```python
from build123d import *

# Parameters (mm, degrees)
SKETCH1_W           = 9.2
SKETCH1_H           = 12
BOSS_EXTRUDE1_DEPTH = 5
SKETCH3_R           = 2
BOSS_EXTRUDE2_DEPTH = 0.5
SKETCH4_R           = 1.5
BOSS_EXTRUDE3_DEPTH = 9.5
CUT_EXTRUDE1_DEPTH  = 9.5
BOSS_EXTRUDE4_DEPTH = 15.5
SKETCH8_W           = 1.5
SKETCH8_H           = 2
CUT_EXTRUDE2_DEPTH  = 1.5
SKETCH9_W           = 0.4
SKETCH9_H           = 1.196619736
BOSS_EXTRUDE5_DEPTH = 1.7
SKETCH10_R          = 2.5
BOSS_EXTRUDE6_DEPTH = 1.5
SKETCH11_R          = 1.675952799
CUT_EXTRUDE3_DEPTH  = 0.5


with BuildPart() as part:
    # Sketch1 → Boss-Extrude1 (new body, symmetric)
    with BuildSketch(Plane(origin=(0, 0, 0), x_dir=(1, 0, 0), z_dir=(0, 1, 0))):
        Rectangle(SKETCH1_W, SKETCH1_H)
    extrude(amount=BOSS_EXTRUDE1_DEPTH, both=True)

    # Sketch3 → Boss-Extrude2 (add)
    with BuildSketch(Plane(origin=(4.6, 0, 0), x_dir=(0, 0, -1), z_dir=(1, 0, 0))):
        Circle(SKETCH3_R)
    extrude(amount=BOSS_EXTRUDE2_DEPTH)

    # Sketch4 → Boss-Extrude3 (add)
    with BuildSketch(Plane(origin=(5.1, 0, 0), x_dir=(0, 0, -1), z_dir=(1, 0, 0))):
        Circle(SKETCH4_R)
    extrude(amount=BOSS_EXTRUDE3_DEPTH)

    # Sketch5 → Cut-Extrude1 (cut)
    with BuildSketch(Plane(origin=(14.6, 0, 0), x_dir=(0, 0, -1), z_dir=(1, 0, 0))):
        with BuildLine():
            Line((-1.118033989, 1), (1.118033989, 1))
            ThreePointArc((1.118033989, 1), (0, 1.5), (-1.118033989, 1))
        make_face()
    extrude(amount=-CUT_EXTRUDE1_DEPTH, mode=Mode.SUBTRACT)

    # Sketch7 → Boss-Extrude4 (add)
    with BuildSketch(Plane.ZY.offset(4.6)):
        with BuildLine():
            Line((-2, -5), (2, -5))
            ThreePointArc((2, -5), (4.828427125, -3.828427125), (6, -1))
            Line((6, -1), (6, 1))
            ThreePointArc((6, 1), (4.828427125, 3.828427125), (2, 5))
            Line((2, 5), (-2, 5))
            ThreePointArc((-2, 5), (-4.828427125, 3.828427125), (-6, 1))
            Line((-6, 1), (-6, -1))
            ThreePointArc((-6, -1), (-4.828427125, -3.828427125), (-2, -5))
        make_face()
    extrude(amount=BOSS_EXTRUDE4_DEPTH)

    # Sketch8 → Cut-Extrude2 (cut)
    with BuildSketch(Plane.ZY.offset(20.1)):
        with Locations((-5.25, 0)):
            Rectangle(SKETCH8_W, SKETCH8_H)
        with Locations((5.25, 0)):
            Rectangle(SKETCH8_W, SKETCH8_H)
    extrude(amount=-CUT_EXTRUDE2_DEPTH, mode=Mode.SUBTRACT)

    # Sketch9 → Boss-Extrude5 (add)
    with BuildSketch(Plane.ZY.offset(20.1)):
        with Locations((-3.5, 0)):
            Rectangle(SKETCH9_W, SKETCH9_H)
        with Locations((3.5, 0)):
            Rectangle(SKETCH9_W, SKETCH9_H)
    extrude(amount=BOSS_EXTRUDE5_DEPTH)

    # Sketch10 → Boss-Extrude6 (add)
    with BuildSketch(Plane.ZY.offset(20.1)):
        Circle(SKETCH10_R)
    extrude(amount=BOSS_EXTRUDE6_DEPTH)

    # Sketch11 → Cut-Extrude3 (cut)
    with BuildSketch(Plane.ZY.offset(21.6)):
        Circle(SKETCH11_R)
    extrude(amount=-CUT_EXTRUDE3_DEPTH, mode=Mode.SUBTRACT)


solid = part.part
```
The model under review builds one solid part; all positions refer to its coordinate system, in mm. A direction names the side the tool comes from. Round coordinates to 2 decimals unless told otherwise and drop trailing zeros. Write each loop counter-clockwise with the first axis right and the second up, starting at its lowest first coordinate (ties: lowest second). Pieces come first, ordered by that corner, then holes. Notation, with made-up numbers: M -9.75,-37.75 L 37.25,-37.75 A26 cw 37.25,-20.75 Z; hole C 62,-6.75 d6. An arc over 180 degrees is marked long. Use CSV: the item, a comma, the result in double quotes. Start each with the question number.
(1) Tool access review of faces 4 (the face through (-21.6, -1, 2)), 5 (the face through (-21.354, -1.636, -0.363)), 6 (the face through (10, 1, 0)), 7 (the face through (4.846, -1.952, 0.434)), 8 (the face through (-19, 1, -5)): name each direction out of +Z, -Z, +X, -X, +Y, -Y from which nothing blocks a thin tool from reaching the whole face with its end or side.
(2) The part is to be moulded in two halves that separate along Y. For faces 1 (the face through (-20.84, -2.44, -0.54)), 2 (the face through (-21, 0, -3.7)), 3 (the face through (-19, -1, 5)), say which applies: +Y half, -Y half, draft (parallel to the pull), parting line (faces both ways), or undercut.
(3) For line 1 along Y through (x, z) = (-21.3, 0); line 2 along X through (y, z) = (2.5, 2.75); line 3 along X through (y, z) = (0, -5), list the stretches that pass through material, from the lowest coordinate up.
(4) Clearance check with flat-ended pins moving along their axes: P1, Ø1, axis at x = -9, y = 3, coming from the -Z side; P2, Ø2, axis at y = -1.5, z = -4, coming from the +X side; P3, Ø0.6, axis at x = -21, y = 0, coming from the +Z side; P4, Ø5, axis at x = -13.5, z = 4.5, coming from the +Y side. State where each tip first meets the part, or that it passes through.
(5) We need section C-C, the plane z = 0. State the section outline as (x, y) points, then the cut area to 3 significant figures.
(6) We need section D-D, the plane y = -3.5. State the section outline as (x, z) points.
(7) We need section A-A, the plane x = -16.5. State the section outline as (y, z) points.
Findings:
1,face 4,"-X, +Y, -Y"
1,face 5,"-X"
1,face 6,"+Z, -Z, +X, +Y"
1,face 7,"+X"
1,face 8,"-Z, -X"
2,face 1,"parting line"
2,face 2,"draft"
2,face 3,"undercut"
3,line 1,"-2.5 to -1.68, 1.68 to 2.5"
3,line 2,"-20.1 to 4.6"
3,line 3,"-18.6 to 4.6"
4,P1,"z = -5.71"
4,P2,"x = 4.6"
4,P3,"z = 3.7"
4,P4,"y = 5"
5,outline,"M -21.6,-2.5 L -20.1,-2.5 L -20.1,-5 L 4.6,-5 L 4.6,-2 L 5.1,-2 L 5.1,-1.5 L 14.6,-1.5 L 14.6,1 L 5.1,1 L 5.1,2 L 4.6,2 L 4.6,5 L -20.1,5 L -20.1,2.5 L -21.6,2.5 L -21.6,1.68 L -21.1,1.68 L -21.1,-1.68 L -21.6,-1.68 Z"
5,area,"279 mm^2"
6,outline,"M -20.1,-5.12 L -4.6,-5.12 L -4.6,-6 L 4.6,-6 L 4.6,6 L -4.6,6 L -4.6,5.12 L -20.1,5.12 Z"
7,outline,"M -5,-2 A4 ccw -1,-6 L 1,-6 A4 ccw 5,-2 L 5,2 A4 ccw 1,6 L -1,6 A4 ccw -5,2 Z"
